Input: part model. Units: mm. Frame: model coordinates. A direction names the side the tool comes from. Round coordinates to 2 decimals unless told otherwise and drop trailing zeros. Loops run counter-clockwise (first coordinate to the right, second up) from the corner with the lowest first, then second, coordinate; pieces in that order, holes last. Notation, with made-up numbers: (72, 47) -> (96, 47) arc R21 cw to (96, 59) -> close; hole circle Ø10 at (34, 43). An arc over 180 degrees is marked (long way). Answer as a JSON object with one key per item and string values. Group by question number.
Item 1: Section query B-B on x = 6.5. Return loops of the section in (y, z).
Item 2: Set-up query: faces 4 (the flat face through (4.338, 4.218, 2.521)), 5 (the flat face through (0, -4, 0)). Return all of +Z, -Z, +X, -X, +Y, -Y with unobstructed straight access to the full face (end or side cutting, diameter ignored); none if empty.
Item 3: Section query A-A on z = 3. Return loops of the section in (x, y).
Item 4: Draft query along Y for faces 1 (the flat face through (-4.876, 4.741, 1.972)), 2 (the flat face through (-3.267, -5.289, 2.188)), 3 (the flat face through (0, -9, 4)). Return one class per face: released by +Y, released by -Y, zero draft, split by the parting line, or undercut.
Item 5: Pin query (flat end, axial travel): pin 1 (2 mm diameter, centred on y = -7.5, z = 1, fed in from -X); pin 2 (8.5 mm diameter, centred on x = 0.5, y = 1.5, fed in from +Z); pin 3 (2 mm diameter, centred on y = -10, z = 1, fed in from +X). Return the tip coordinate at first contact, or that it passes through.
Item 6: Material intervals for line 1 (Z direction, x = 3.25, y = 4.75); line 2 (Y direction, x = -1.75, z = 2.7); line 3 (Y direction, x = -7.75, z = 2), sorted ascending. Write a range as [from, to].
Item 7: Section query C-C on z = 1.55. Return loops of the section in (x, y).
Item 8: Section query D-D on y = 6.25. Return loops of the section in (x, z).
from build123d import *

# Parameters (mm, degrees)
F0_W        = 13.6
F0_H        = 13.6
F1_DEPTH    = 4
F2_W        = 12.1
F2_H        = 12.1
F3_DEPTH    = 3
F5_ANGLE    = 45
F7_DEPTH    = 4
F8_T1_DEPTH = 35.422011596
F8_T3_DEPTH = 35.422011596


# Not quite as in the source:
# - a fillet or chamfer that OpenCascade refuses, or shapes differently, is made with other operations: its cross-section is extruded or revolved along the edge and cut away or added


with BuildPart() as f1:
    # F0 (on Top) → F1 (new body)
    with BuildSketch(Plane.XY):
        Rectangle(F0_W, F0_H)
    extrude(amount=F1_DEPTH)

    # F2 (on face) → F3 (cut)
    with BuildSketch(Plane.XY.offset(4)):
        Rectangle(F2_W, F2_H)
    extrude(amount=-F3_DEPTH, mode=Mode.SUBTRACT)


with BuildPart() as f1_1:
    # F5: moved
    add(f1.part.rotate(Axis((0, 0, 16.5512096137), (0, 0, 1)), F5_ANGLE))

    # F6 (on face) → F7 (join)
    with BuildSketch(Plane(origin=(0, 0, 0), x_dir=(1, 0, 0), z_dir=(0, 0, -1))):
        Polygon((0, 9.6166522241), (9.6166522241, 0), (0, 17.527025193), (-9.6166522241, 0), align=None)
    extrude(amount=-F7_DEPTH)

    # F8: chamfer of 3 on 2 edges, made by hand

    # F8_s2 → F8_t1 (cut)
    with BuildSketch(Plane(origin=(5.9363165934, 10.8193546008, 0), x_dir=(0, 0, 1), z_dir=(-0.4810270984, -0.8767057263, 0))):
        Polygon((4, -5.4309740729), (1, -8.4309740729), (4, -8.4309740729), align=None)
    extrude(amount=F8_T1_DEPTH, mode=Mode.SUBTRACT)

    # F8_s4 → F8_t3 (cut)
    with BuildSketch(Plane(origin=(11.1026308657, -20.2353258031, 0), x_dir=(0, 0, 1), z_dir=(-0.4810270984, 0.8767057263, 0))):
        Polygon((1, -8.4309740729), (4, -5.4309740729), (4, -8.4309740729), align=None)
    extrude(amount=F8_T3_DEPTH, mode=Mode.SUBTRACT)


solid = f1_1.part
Solved:
{
 "1": {"outline": "(-5.68, 0) -> (3.12, 0) -> (3.12, 4) -> (2.06, 4) -> (2.06, 1) -> (-2.06, 1) -> (-2.06, 2.74) -> (-5.68, 1) -> close"},
 "2": {"face 4": "+Z", "face 5": "-Z, +X, -X, +Y, -Y"},
 "3": {"outline": "(-8.14, 1.47) -> (-7.77, 0.79) -> (0, 8.56) -> (7.77, 0.79) -> (8.14, 1.47) -> (0, 9.62) -> close; (-5.85, -2.7) -> (0, -13.37) -> (5.85, -2.7) -> (0, -8.56) -> close"},
 "4": {"face 1": "released by +Y", "face 2": "undercut", "face 3": "zero draft"},
 "5": {"pin 1": "x = -6.05", "pin 2": "z = 1", "pin 3": "x = 4.68"},
 "6": {"line 1": "[0, 1]", "line 2": "[-10.8, -6.81], [6.81, 7.87]", "line 3": "[-1.32, -0.81], [0.81, 1.87]"},
 "7": {"outline": "(-9.21, 0.41) -> (0, -16.38) -> (9.21, 0.41) -> (0, 9.62) -> close; hole (-8.56, 0) -> (0, -8.56) -> (8.56, 0) -> (0, 8.56) -> close"},
 "8": {"outline": "(-3.37, 0) -> (3.37, 0) -> (3.37, 4) -> (2.31, 4) -> (2.31, 1) -> (-2.31, 1) -> (-2.31, 4) -> (-3.37, 4) -> close"}
}
